Answer from the drawing. Dimensions are ordinates in mm from the lowest x, y and z of the part. A direction names the side the tool comes from. Round coordinates to 2 decimals unless told otherwise and drop trailing zeros. Order: outer loops, then holes, each group sorted by start corner. A loop starts at its lowest first (then second) coordinate and runs counter-clockwise, first axis right, second up. Notation, with made-up numbers: M 49,78.5 L 95,78.5 A32 ccw 95,116.5 Z; hole C 2.25,31 d2. An arc over 180 degrees is marked long. Write item = value, one per line. Start each with the question number.
(1) A cutting plane is placed at B-B, the plane z = 8. Determine the outline of the cut face in (x, y).
(2) A cutting plane is placed at C-C, the plane y = 1.5. Determine the outline of the cut face in (x, z).
(3) A cutting plane is placed at D-D, the plane z = 13.5. Determine the outline of the cut face in (x, y), and give its area (3 significant figures).
(4) For a pull along Y with two mould halves and no side action, classify the marked faces 1, 2, 3 and 4 as released by +Y, released by -Y, zero draft, split by the parting line, or undercut.
(5) Each of these flat-tipped pins is pushed along its axis until it touches: pin 1 (8 mm diameter, centred on y = 7, z = 13, fed in from +X); pin 2 (4.5 mm diameter, centred on x = 14.5, y = 8, fed in from -Z). Where does it stop, or does it pass through?
(6) A cutting plane is placed at A-A, the plane y = 3.5. Determine the outline of the cut face in (x, z) (1 decimal).
(7) Straight lines are drawn through the part: probe 1 along Z at (x, y) = (9.25, 5.5); probe 2 along X at (y, z) = (7.5, 7.25); probe 3 along Z at (x, y) = (19.5, 11.5). For each, find the intervals that lie inside material, in ascending order. Write a range as from..to.
(8) Which of the six approach directions +Z, -Z, +X, -X, +Y, -Y give full straight-line access (tool end or side, diameter ignored) to the marked faces 5, 6 and 7?
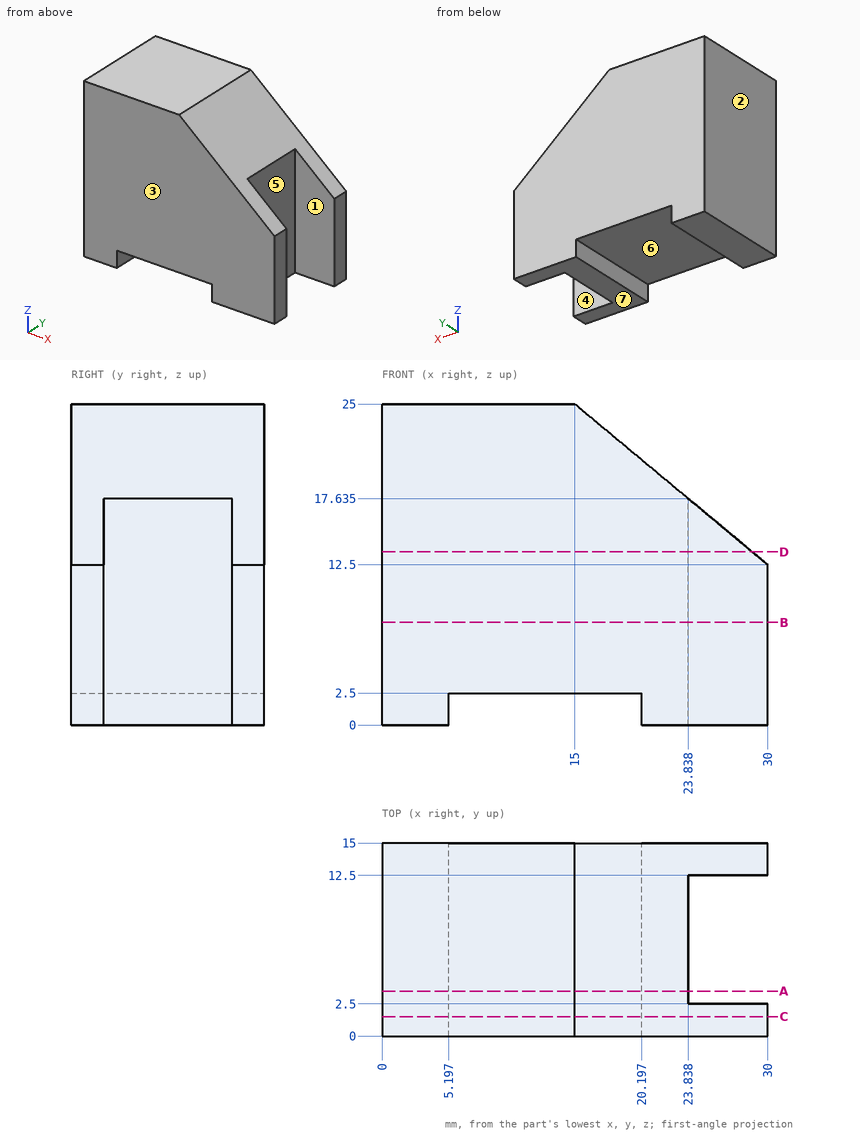
Reported:
q1.outline = M 0,0 L 30,0 L 30,2.5 L 23.84,2.5 L 23.84,12.5 L 30,12.5 L 30,15 L 0,15 Z
q2.outline = M 0,0 L 5.2,0 L 5.2,2.5 L 20.2,2.5 L 20.2,0 L 30,0 L 30,12.5 L 15,25 L 0,25 Z
q3.outline = M 0,0 L 28.8,0 L 28.8,2.5 L 23.84,2.5 L 23.84,12.5 L 28.8,12.5 L 28.8,15 L 0,15 Z
q3.area = 382 mm²
q4.face_1 = undercut
q4.face_2 = zero draft
q4.face_3 = released by -Y
q4.face_4 = undercut
q5.pin_1 = 23.84
q5.pin_2 = 2.5
q6.outline = M 0,0 L 5.2,0 L 5.2,2.5 L 20.2,2.5 L 20.2,0 L 23.8,0 L 23.8,17.6 L 15,25 L 0,25 Z
q7.probe_1 = 2.5..25
q7.probe_2 = 0..23.84
q7.probe_3 = 2.5..21.25
q8.face_5 = +Z, -Z, +X
q8.face_6 = -Z, +Y, -Y
q8.face_7 = -Z, +X, -X, +Y, -Y
